Design review of the part built by this model. Coordinates are the model's own, in mm. Round coordinates to 2 decimals unless told otherwise and drop trailing zeros. Order: outer loops, then holes, each group sorted by start corner. A loop starts at its lowest first (then second) coordinate and runs counter-clockwise, first axis right, second up. Notation, with made-up numbers: (86, 1) - (112, 1) arc R23 ccw to (112, 26) - close; hole circle Ø7 at (65.25, 34). An arc over 180 degrees is marked (long way). Write item = value, one per line.
from build123d import *

# Parameters (mm, degrees)
SKETCH1_W           = 207
SKETCH1_H           = 114.5
SKETCH1_W_2         = 187
SKETCH1_H_2         = 40
SKETCH1_W_3         = 191
SKETCH1_H_3         = 5.5
SKETCH1_R           = 1.6
SKETCH1_W_4         = 4
SKETCH1_H_4         = 11.5
BOSS_EXTRUDE1_DEPTH = 3.2
SKETCH1_3_W         = 207
SKETCH1_3_H         = 114.5
SKETCH1_3_W_2       = 187
SKETCH1_3_H_2       = 40
SKETCH1_3_R         = 1.6
SKETCH1_3_W_3       = 4
SKETCH1_3_H_3       = 11.5
BOSS_EXTRUDE2_DEPTH = 3


with BuildPart() as part:
    # Sketch1 → Boss-Extrude1 (new body)
    with BuildSketch(Plane(origin=(0, 0, 0), x_dir=(1, 0, 0), z_dir=(0, 1, 0))):
        Rectangle(SKETCH1_W, SKETCH1_H)
        with Locations((0, 25.75)):
            Rectangle(SKETCH1_W_2, SKETCH1_H_2, mode=Mode.SUBTRACT)
        Polygon((93.5, 2.75), (95.5, 2.75), (95.5, -2.75), (-95.5, -2.75), (-95.5, 2.75), align=None, mode=Mode.SUBTRACT)
        with Locations((0, -25.75)):
            Rectangle(SKETCH1_W_2, SKETCH1_H_2, mode=Mode.SUBTRACT)
        with Locations((0, -51.5)):
            Rectangle(SKETCH1_W_3, SKETCH1_H_3, mode=Mode.SUBTRACT)
        with Locations((0, 51.5)):
            Rectangle(SKETCH1_W_3, SKETCH1_H_3, mode=Mode.SUBTRACT)
        with Locations((-99.5, -51.5)):
            Circle(SKETCH1_R, mode=Mode.SUBTRACT)
        with Locations((-99.5, 0)):
            Rectangle(SKETCH1_W_4, SKETCH1_H_4, mode=Mode.SUBTRACT)
        with Locations((-99.5, 51.5)):
            Circle(SKETCH1_R, mode=Mode.SUBTRACT)
        with Locations((99.5, 51.5)):
            Circle(SKETCH1_R, mode=Mode.SUBTRACT)
        with Locations((99.5, -51.5)):
            Circle(SKETCH1_R, mode=Mode.SUBTRACT)
        with Locations((99.5, 0)):
            Rectangle(SKETCH1_W_4, SKETCH1_H_4, mode=Mode.SUBTRACT)
    extrude(amount=BOSS_EXTRUDE1_DEPTH)

    # Sketch1_3 → Boss-Extrude2 (add)
    with BuildSketch(Plane(origin=(0, 0, 0), x_dir=(1, 0, 0), z_dir=(0, 1, 0))):
        Rectangle(SKETCH1_3_W, SKETCH1_3_H)
        with Locations((0, 25.75)):
            Rectangle(SKETCH1_3_W_2, SKETCH1_3_H_2, mode=Mode.SUBTRACT)
        with Locations((0, -25.75)):
            Rectangle(SKETCH1_3_W_2, SKETCH1_3_H_2, mode=Mode.SUBTRACT)
        with Locations((-99.5, -51.5)):
            Circle(SKETCH1_3_R, mode=Mode.SUBTRACT)
        with Locations((-99.5, 0)):
            Rectangle(SKETCH1_3_W_3, SKETCH1_3_H_3, mode=Mode.SUBTRACT)
        with Locations((-99.5, 51.5)):
            Circle(SKETCH1_3_R, mode=Mode.SUBTRACT)
        with Locations((99.5, 51.5)):
            Circle(SKETCH1_3_R, mode=Mode.SUBTRACT)
        with Locations((99.5, 0)):
            Rectangle(SKETCH1_3_W_3, SKETCH1_3_H_3, mode=Mode.SUBTRACT)
        with Locations((99.5, -51.5)):
            Circle(SKETCH1_3_R, mode=Mode.SUBTRACT)
    extrude(amount=-BOSS_EXTRUDE2_DEPTH)


solid = part.part
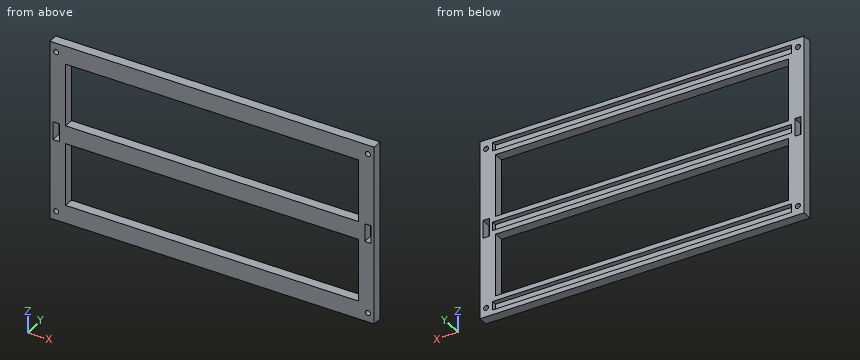
Item 1: Take a section at A-A, the plane z = 23.5. State the section outline as (x, y) points, and give its area (3 significant figures).
Data:
outline = (-103.5, -3) - (-93.5, -3) - (-93.5, 3.2) - (-103.5, 3.2) - close; (93.5, -3) - (103.5, -3) - (103.5, 3.2) - (93.5, 3.2) - close
area = 124 mm2
Item 2: Take a section at D-D, the plane y = -1.25. Count the separate pieces of the cut face and the enclosed holes in it, and give its area (3 significant figures).
Data:
separate_pieces = 1
enclosed_holes = 8
area = 8,620 mm2
Item 3: Take a section at C-C, the plane x = -66.5. State the section outline as (y, z) points.
Data:
outline = (-3, -57.25) - (3.2, -57.25) - (3.2, -54.25) - (0, -54.25) - (0, -48.75) - (3.2, -48.75) - (3.2, -45.75) - (-3, -45.75) - close; (-3, -5.75) - (3.2, -5.75) - (3.2, -2.75) - (0, -2.75) - (0, 2.75) - (3.2, 2.75) - (3.2, 5.75) - (-3, 5.75) - close; (-3, 45.75) - (3.2, 45.75) - (3.2, 48.75) - (0, 48.75) - (0, 54.25) - (3.2, 54.25) - (3.2, 57.25) - (-3, 57.25) - close
Item 4: For line 1 along Z through (x, y) = (77, -1.75); line 2 along X through (y, z) = (1.5, -51.5); line 3 along Z through (x, y) = (-99.5, 1.5), list the stretches that pass through material, from the lowest coordinate up. Write a range as [from, to].
Data:
line_1 = [-57.25, -45.75], [-5.75, 5.75], [45.75, 57.25]
line_2 = [-103.5, -101.1], [-97.9, -95.5], [95.5, 97.9], [101.1, 103.5]
line_3 = [-57.25, -53.1], [-49.9, -5.75], [5.75, 49.9], [53.1, 57.25]
Item 5: Insertion check: P1, Ø3, axis at x = -99.5, z = -51.5, coming from the +Y side; P2, Ø5, axis at x = 99.5, z = 51.5, coming from the +Y side. Each pin has a flat end and moves straight along its axis. Give the tip position at first contact, or say it passes through.
Data:
P1 = through
P2 = 3.2
Item 6: Take a section at B-B, the plane z = 0. State the section outline as (x, y) points.
Data:
outline = (-103.5, -3) - (-101.5, -3) - (-101.5, 3.2) - (-103.5, 3.2) - close; (-97.5, -3) - (97.5, -3) - (97.5, 3.2) - (95.5, 3.2) - (95.5, 0) - (-95.5, 0) - (-95.5, 3.2) - (-97.5, 3.2) - close; (101.5, -3) - (103.5, -3) - (103.5, 3.2) - (101.5, 3.2) - close
